from build123d import *

# Parameters (mm, degrees)
SKETCH_1_W               = 25
SKETCH_1_H               = 25
EXTRUDE_1_DEPTH          = 100
PATTERN_LINEAR_1_COUNT   = 2
PATTERN_LINEAR_1_PITCH   = 100
PATTERN_LINEAR_1_2_COUNT = 2
PATTERN_LINEAR_1_2_PITCH = 100
SKETCH_2_W               = 125
SKETCH_2_H               = 125
EXTRUDE_2_DEPTH          = 10
SKETCH_3_W               = 15
SKETCH_3_H               = 20
EXTRUDE_3_DEPTH          = 200
EXTRUDE_4_REACH          = 349.536
SKETCH_4_W               = 20
SKETCH_4_H               = 20
PATTERN_LINEAR_2_COUNT   = 2
PATTERN_LINEAR_2_PITCH   = 90
SKETCH_5_W               = 15
SKETCH_5_H               = 20
EXTRUDE_5_DEPTH          = 100
EXTRUDE_6_REACH          = 392.872
SKETCH_6_W               = 20
SKETCH_6_H               = 14.103809958
CUT_EXTRUDE_1_REACH      = 389.016
SKETCH_7_W               = 19.107608913
SKETCH_7_H               = 7.486425105
SKETCH_8_W               = 72.938493455
SKETCH_8_H               = 19.454848412
EXTRUDE_7_DEPTH          = 5
SKETCH_9_W               = 66.78878025
SKETCH_9_H               = 20
EXTRUDE_8_DEPTH          = 5
MIRROR_1_COPY_1_REACH    = 349.536
MIRROR_1_COPY_1_SKETCH_W = 20
MIRROR_1_COPY_1_SKETCH_H = 20
EXTRUDE_9_DEPTH          = 10
EXTRUDE_9_DEPTH_BACK     = 30
SKETCH_10_W              = 19.107608913
SKETCH_10_H              = 6.617384853
EXTRUDE_10_DEPTH         = 10
EXTRUDE_10_DEPTH_BACK    = 30
SKETCH_11_W              = 19.107608913
SKETCH_11_H              = 6.617384853


with BuildPart() as part:
    # Sketch 1 → Extrude 1 (new body)
    with BuildSketch(Plane(origin=(0, 0, 0), x_dir=(1, 0, 0), z_dir=(0, 1, 0))):
        Rectangle(SKETCH_1_W, SKETCH_1_H)
    extrude(amount=EXTRUDE_1_DEPTH)


with BuildPart() as pattern_linear_1_1:
    # Pattern Linear 1: pattern copy
    add(part.part.moved(Location(Vector(0, 0, 1) * (1 * PATTERN_LINEAR_1_PITCH))))


with BuildPart() as pattern_linear_1_2_1:
    # Pattern Linear 1 2: pattern copy
    add(part.part.moved(Location(Vector(1, 0, 0) * (1 * PATTERN_LINEAR_1_2_PITCH))))


with BuildPart() as pattern_linear_1_2_2:
    # Pattern Linear 1 2: pattern copy
    add(pattern_linear_1_1.part.moved(Location(Vector(1, 0, 0) * (1 * PATTERN_LINEAR_1_2_PITCH))))


with BuildPart() as part_1:
    add(part.part)

    add(pattern_linear_1_1.part)  # Extrude 2 merges Pattern Linear 1_1

    add(pattern_linear_1_2_1.part)  # Extrude 2 merges Pattern Linear 1 2_1

    add(pattern_linear_1_2_2.part)  # Extrude 2 merges Pattern Linear 1 2_2
    # Sketch 2 → Extrude 2 (add)
    with BuildSketch(Plane(origin=(0, 100, 0), x_dir=(1, 0, 0), z_dir=(0, 1, 0))):
        with Locations((50, -50)):
            Rectangle(SKETCH_2_W, SKETCH_2_H)
    extrude(amount=EXTRUDE_2_DEPTH)

    # Sketch 3 → Extrude 3 (add)
    with BuildSketch(Plane.XY.offset(112.5)):
        with Locations((0, 100)):
            Rectangle(SKETCH_3_W, SKETCH_3_H)
        with Locations((100, 100)):
            Rectangle(SKETCH_3_W, SKETCH_3_H)
    extrude_3 = extrude(amount=EXTRUDE_3_DEPTH)

    # Sketch 4 → Extrude 4 (add, up to next)
    with BuildSketch(Plane(origin=(7.5, 0, 0), x_dir=(0, 0, -1), z_dir=(1, 0, 0)), mode=Mode.PRIVATE) as extrude_4_sk1:
        with Locations((-212.5, 100)):
            Rectangle(SKETCH_4_W, SKETCH_4_H)
    extrude_4_tool1 = extrude(extrude_4_sk1.sketch, amount=EXTRUDE_4_REACH, mode=Mode.PRIVATE) - part_1.part
    extrude_4 = extrude_4_tool1.solids().sort_by_distance((7.5, 100, 212.5))[0]
    add(extrude_4)

    # Pattern Linear 2: Extrude 4 ×2
    with Locations(*[(0, 0, i * PATTERN_LINEAR_2_PITCH) for i in range(1, PATTERN_LINEAR_2_COUNT)]):
        add(extrude_4)

    # Sketch 5 → Extrude 5 (add)
    with BuildSketch(Plane(origin=(0, 110, 0), x_dir=(1, 0, 0), z_dir=(0, 1, 0))):
        with Locations((100, -302.5)):
            Rectangle(SKETCH_5_W, SKETCH_5_H)
        with Locations((0, -302.5)):
            Rectangle(SKETCH_5_W, SKETCH_5_H)
    extrude_5 = extrude(amount=EXTRUDE_5_DEPTH)

    # Sketch 6 → Extrude 6 (add, up to next)
    with BuildSketch(Plane(origin=(7.5, 0, 0), x_dir=(0, 0, -1), z_dir=(1, 0, 0)), mode=Mode.PRIVATE) as extrude_6_sk1:
        with Locations((-302.5, 202.948095021)):
            Rectangle(SKETCH_6_W, SKETCH_6_H)
    extrude_6_tool1 = extrude(extrude_6_sk1.sketch, amount=EXTRUDE_6_REACH, mode=Mode.PRIVATE) - part_1.part
    extrude_6 = extrude_6_tool1.solids().sort_by_distance((7.5, 202.948095, 302.5))[0]
    add(extrude_6)

    # Sketch 7 → Cut-Extrude 1 (cut, up to next)
    with BuildSketch(Plane(origin=(0, 0, 292.5), x_dir=(-1, 0, 0), z_dir=(0, 0, -1)), mode=Mode.PRIVATE) as cut_extrude_1_sk1:
        with Locations((-54.190265113, 206.256787448)):
            Rectangle(SKETCH_7_W, SKETCH_7_H)
    cut_extrude_1_tool1 = extrude(cut_extrude_1_sk1.sketch, amount=-CUT_EXTRUDE_1_REACH, mode=Mode.PRIVATE) & part_1.part
    cut_extrude_1 = cut_extrude_1_tool1.solids().sort_by_distance((54.190265, 206.256787, 292.5))[0]
    add(cut_extrude_1, mode=Mode.SUBTRACT)

    # Sketch 8 → Extrude 7 (add)
    with BuildSketch(Plane(origin=(0, 210, 0), x_dir=(1, 0, 0), z_dir=(0, 1, 0))):
        with Locations((-28.969246727, -302.227424206)):
            Rectangle(SKETCH_8_W, SKETCH_8_H)
    extrude_7 = extrude(amount=EXTRUDE_7_DEPTH)

    # Sketch 9 → Extrude 8 (add)
    with BuildSketch(Plane(origin=(0, 210, 0), x_dir=(1, 0, 0), z_dir=(0, 1, 0))):
        with Locations((125.894390125, -302.5)):
            Rectangle(SKETCH_9_W, SKETCH_9_H)
    extrude_8 = extrude(amount=EXTRUDE_8_DEPTH)

    # Mirror 1: Extrude 3, Extrude 4, Extrude 5, Extrude 6, Cut-Extrude 1, Extrude 7, Extrude 8 across plane
    add(extrude_3.mirror(Plane.XY.offset(50)))
    add(extrude_4.mirror(Plane.XY.offset(50)))
    add(extrude_5.mirror(Plane.XY.offset(50)))
    add(extrude_6.mirror(Plane.XY.offset(50)))
    add(cut_extrude_1.mirror(Plane.XY.offset(50)), mode=Mode.SUBTRACT)
    add(extrude_7.mirror(Plane.XY.offset(50)))
    add(extrude_8.mirror(Plane.XY.offset(50)))

    # Mirror 1 copy 1 sketch → Mirror 1 copy 1 (add, up to next)
    with BuildSketch(Plane(origin=(7.5, 0, 10), x_dir=(0, 0, 1), z_dir=(1, 0, 0)), mode=Mode.PRIVATE) as mirror_1_copy_1_sk1:
        with Locations((-212.5, -100)):
            Rectangle(MIRROR_1_COPY_1_SKETCH_W, MIRROR_1_COPY_1_SKETCH_H)
    mirror_1_copy_1_tool1 = extrude(mirror_1_copy_1_sk1.sketch, amount=MIRROR_1_COPY_1_REACH, mode=Mode.PRIVATE) - part_1.part
    add(mirror_1_copy_1_tool1.solids().sort_by_distance((7.5, 100, -202.5))[0])

    # Sketch 10 → Extrude 9 (add, two sides: drawn at the far end of the back side and taken through both)
    with BuildSketch(Plane.XY.offset(312.5).offset(-EXTRUDE_9_DEPTH_BACK)):
        with Locations((54.190265113, 199.204882468)):
            Rectangle(SKETCH_10_W, SKETCH_10_H)
    extrude(amount=EXTRUDE_9_DEPTH + EXTRUDE_9_DEPTH_BACK)

    # Sketch 11 → Extrude 10 (add, two sides: drawn at the far end of the back side and taken through both)
    with BuildSketch(Plane.XY.offset(-192.5).offset(-EXTRUDE_10_DEPTH_BACK)):
        with Locations((54.190265113, 199.204882468)):
            Rectangle(SKETCH_11_W, SKETCH_11_H)
    extrude(amount=EXTRUDE_10_DEPTH + EXTRUDE_10_DEPTH_BACK)


solid = part_1.part
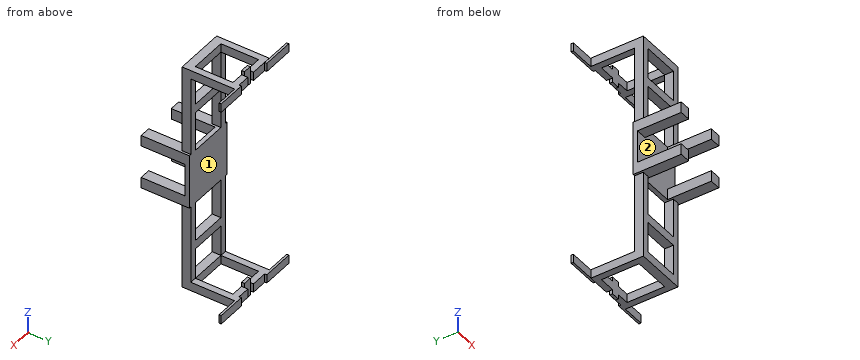
CAD build for the part. Positions are in the model's coordinates, mm. Face numbers are marked on the shaded views. Round coordinates to 2 decimals unless told otherwise and drop trailing zeros. Write each loop counter-clockwise with the first axis right and the second up, starting at its lowest first coordinate (ties: lowest second). Pieces come first, ordered by that corner, then holes.
(1) Slice it at A-A, the plane y = 57.5. Write the cut outline in (x, z).
(2) Slice it at B-B, the plane z = 272.5. Write the cut outline in (x, y).
(3) Slice it at D-D, the plane x = 20.5. Write the cut outline in (y, z).
(4) Mould opens along X. For the marked faces 1 and 2 say: pulls with the +X half, pulls with the -X half, needs draft (parallel to the pull), parting line crosses it, or undercut.
(5) Drop flat-ended pins along their axis: P1, Ø22, axis at y = 163.5, z = -204.5, coming from the -X side; P2, Ø12, axis at x = 65, z = -200, coming from the -Y side; P3, Ø8, axis at x = 96, y = 187, coming from the +Z side. Give the stop position or say it passes through.
(6) Slice it at C-C, the plane x = 118. Write the cut outline in (y, z), and give its area (3 significant figures).
(7) Probe line 1 along X through (y, z) = (106.5, -175); line 2 along Z through (x, y) = (-5.5, 200); line 3 along Y through (x, z) = (86, -113). List the from-to ranges inside material, lowest first.
From the geometry:
1. outline: (-12.5, -12.5) - (12.5, -12.5) - (12.5, 12.5) - (-12.5, 12.5) - close; (-12.5, 87.5) - (12.5, 87.5) - (12.5, 112.5) - (-12.5, 112.5) - close; (87.5, -12.5) - (112.5, -12.5) - (112.5, 12.5) - (87.5, 12.5) - close; (87.5, 87.5) - (112.5, 87.5) - (112.5, 112.5) - (87.5, 112.5) - close
2. outline: (-7.5, 90) - (7.5, 90) - (7.5, 110) - (-7.5, 110) - close; (92.5, 90) - (107.5, 90) - (107.5, 110) - (92.5, 110) - close
3. outline: (90, -212.5) - (110, -212.5) - (110, -192.5) - (90, -192.5) - close; (90, -122.5) - (110, -122.5) - (110, -102.5) - (90, -102.5) - close; (90, 202.5) - (110, 202.5) - (110, 222.5) - (90, 222.5) - close; (90, 292.5) - (110, 292.5) - (110, 312.5) - (90, 312.5) - close; (100, -12.5) - (110, -12.5) - (110, 112.5) - (100, 112.5) - close; (195.9, -212.5) - (210, -212.5) - (210, -192.5) - (195.9, -192.5) - close; (195.9, 292.5) - (210, 292.5) - (210, 312.5) - (195.9, 312.5) - close
4. face 1: needs draft
4. face 2: undercut
5. P1: stops at x = -7.5
5. P2: stops at y = 90
5. P3: stops at z = 312.5
6. outline: (210, -212.5) - (215, -212.5) - (215, -192.5) - (210, -192.5) - close; (210, 292.5) - (215, 292.5) - (215, 312.5) - (210, 312.5) - close
6. area: 200 mm2
7. line 1: x = -7.5 to 7.5, 92.5 to 107.5
7. line 2: z = -212.5 to -192.5, 292.5 to 312.5
7. line 3: y = 90 to 110
